The model under review builds one solid part; all positions refer to its coordinate system, in mm. Face numbers are marked on the shaded views. Coordinates: 2 decimals unless noted, no trailing zeros. Write each loop counter-clockwise with the first axis right and the second up, starting at its lowest first coordinate (ties: lowest second). Pieces come first, ordered by that corner, then holes. Notation, with made-up numbers: (1, -28.75) - (17, -28.75) arc R25 cw to (17, 5.25) - close; hole circle Ø2 at (25, -16). An arc over 180 degrees is marked (long way). Return JSON: item names as keys, results as strings. Group by question number.
(1) Draft analysis for pull direction X (two halves, no side actions). For the marked faces 1, 2 and 3, state which applies: released by +X, released by -X, zero draft, split by the parting line, or undercut.
(2) We need section A-A on x = 30. State the section outline as (y, z) points, then the cut area to 3 significant figures.
(3) For pin 1 Ø16 at (x, z) = (30, -20) entering from -Y, flat-tipped, find the tip position at first contact; note if it passes through.
(4) We need section B-B on z = -20. State the section outline as (x, y) points.
(5) We need section C-C on y = 18.75. State the section outline as (x, z) points.
(6) To check wall thickness, follow L1, parallel to Z at x = 30, y = 15.75; L2, parallel to Z at x = 29, y = 3.5; L3, parallel to X at y = 7.5, z = -18. State the ranges of each line that lie inside material, in increasing order. Write a range as from..to.
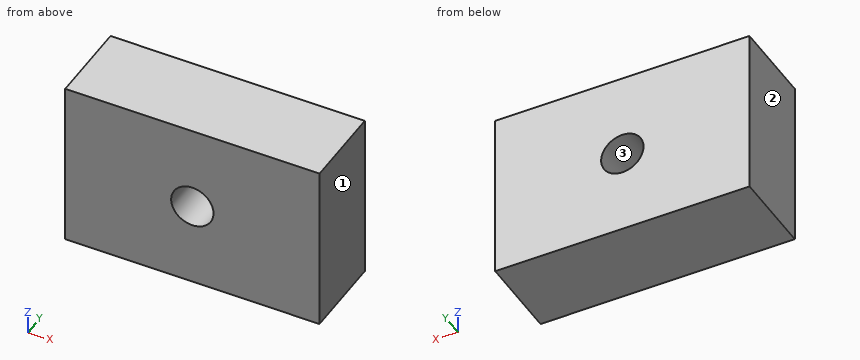
Autodesk Fusion 360 part; units mm, degrees
sketch "草图1" plane through (0, 0, 0) normal (0, 1, 0) x (1, 0, 0)
  line L0 (0, 0) -> (60, 0)
  line L1 (60, 0) -> (60, 40)
  line L2 (60, 40) -> (0, 40)
  line L3 (0, 40) -> (0, 0)
extrude "拉伸1" add sketch "草图1" along normal blind 20
sketch "草图2" plane through (0, 20, 0) normal (0, 1, 0) x (-1, 0, 0)
  line L0 (0, -40) -> (0, 0)
  line L1 (0, 0) -> (-60, 0)
  line L2 (-60, 0) -> (-60, -40)
  line L3 (-60, -40) -> (0, -40)
  line L4 (0, 0) -> (-60, -40) construction
  line L5 (0, -40) -> (-60, 0) construction
  circle A0 centre (-30, -20) radius 5
  dimension "d3" = 10
extrude "拉伸2" cut sketch "草图2" against normal through all contours A0
Ans:
{
 "1": {"face 1": "released by +X", "face 2": "released by -X", "face 3": "undercut"},
 "2": {"outline": "(0, -40) - (20, -40) - (20, -25) - (0, -25) - close; (0, -15) - (20, -15) - (20, 0) - (0, 0) - close", "area": "600 mm²"},
 "3": {"pin 1": "y = 0"},
 "4": {"outline": "(0, 0) - (25, 0) - (25, 20) - (0, 20) - close; (35, 0) - (60, 0) - (60, 20) - (35, 20) - close"},
 "5": {"outline": "(0, -40) - (60, -40) - (60, 0) - (0, 0) - close; hole circle Ø10 at (30, -20)"},
 "6": {"L1": "-40..-25, -15..0", "L2": "-40..-24.9, -15.1..0", "L3": "0..25.42, 34.58..60"}
}
